Design review of the part built by this model. Coordinates are the model's own, in mm. A direction names the side the tool comes from. Give positions to 0.01 mm unless a question says otherwise; leave off trailing zeros. Loops run counter-clockwise (first coordinate to the right, second up) from the corner with the lowest first, then second, coordinate; pieces in that order, holes last.
Autodesk Inventor part; units mm, degrees
ref_plane "ABDECKKAPPE_XY" through (0, 0, 158) normal (0, 0, 1) x (1, 0, 0)
ref_plane "ABDECKKAPPE_YZ" through (0, 0, 158) normal (1, 0, 0) x (0, 1, 0)
ref_plane "ABDECKKAPPE_ZX" through (0, 0, 158) normal (0, 1, 0) x (0, 0, 1)
sketch "Sketch_1" plane through (0, 0, 0) normal (1, 0, 0) x (0, 0, -1)
  line L0 (0, 0) -> (-184, 0)
  line L1 (-184, 19.7) -> (-184, 17.75)
  line L2 (-184, 17.75) -> (-183.5, 17.25)
  line L3 (-183.5, 17.25) -> (-165, 17.25)
  line L4 (-165, 17.25) -> (-164.2489, 16)
  line L5 (-164.2489, 16) -> (-22.7511, 16)
  line L6 (-22.7511, 16) -> (-22, 17.25)
  line L7 (-22, 17.25) -> (-3, 17.25)
  line L8 (-3, 17.25) -> (-3, 18.5)
  line L9 (-3, 18.5) -> (0, 18.5)
  line L10 (0, 18.5) -> (0, 20)
  line L11 (0, 20) -> (-162.7709, 20)
  arc A0 (-163.2291, 20) -> (-162.7709, 20) centre (-163, 20.1) ccw
  line L12 (-163.2291, 20) -> (-183.7, 20)
  line L13 (-183.7, 20) -> (-184, 19.7)
revolve "Revolution1" add sketch "Sketch_1" angle 360 about axis through (0, 0, 0) along (0, 0, -1)
ref_plane "ABDECKKAPPE_XY" through (0, 0, 158) normal (0, 0, 1) x (1, 0, 0)
ref_plane "ABDECKKAPPE_YZ" through (0, 0, 158) normal (1, 0, 0) x (0, 1, 0)
ref_plane "ABDECKKAPPE_ZX" through (0, 0, 158) normal (0, 1, 0) x (0, 0, 1)
ref_plane "SCHUBSTANGE_XY" through (0, 0, 184) normal (0, 0, -1) x (1, 0, 0)
ref_plane "SCHUBSTANGE_YZ" through (0, 0, 184) normal (1, 0, 0) x (0, -1, 0)
ref_plane "SCHUBSTANGE_ZX" through (0, 0, 184) normal (0, -1, 0) x (0, 0, -1)
properties part number "SLZ_63_Schubstange#_274.5_1001"
Q1. Draft analysis for pull direction X (two halves, no side actions). For faces 3 (the face through (19.524, -4.336, 173.608)), 4 (the face through (-18, 6, 0)), 5 (the face through (5.181, 16.453, 174.12)), state which applies: pulls with the +X half, pulls with the -X half, needs draft (parallel to the pull), parting line crosses it, or undercut.
Results:
face 3: parting line crosses it
face 4: needs draft
face 5: undercut
Q2. Take a section at D-D (z = 25). Give the boundary of the cut face in (x, y).
Results:
outline: circle Ø40 at (0, 0); hole circle Ø32 at (0, 0)
Q3. Wall thickness on line 1 (X direction, y = 0, z = 51); line 2 (X direction, y = -0.5, z = 174); line 3 (Y direction, x = 8, z = 64): over which ranges is each line inside the solid? List them lowest first.
Results:
line 1: x = -20 to -16, 16 to 20
line 2: x = -19.99 to -17.24, 17.24 to 19.99
line 3: y = -18.33 to -13.86, 13.86 to 18.33
Q4. Insertion check: pin 1 (1.5 mm diameter, centred on x = -6.5, z = 73.5, fed in from +Y); pin 2 (8 mm diameter, centred on y = 7.5, z = 108.5, fed in from -X); pin 3 (6 mm diameter, centred on y = 3, z = 135, fed in from +X). Each pin has a flat end and moves straight along its axis. Give the tip position at first contact, or say it passes through.
Results:
pin 1: stops at y = 19.16
pin 2: stops at x = -19.69
pin 3: stops at x = 20
Q5. Tool access review of faces 1 (the face through (19.524, -4.336, 82.525)), 2 (the face through (17, 5, 3)): name each direction out of +Z, -Z, +X, -X, +Y, -Y from which nothing blocks a thin tool from reaching the whole face with its end or side.
Results:
face 1: +Z, -Z
face 2: -Z
Q6. Take a section at A-A (x = 0). Give the boundary of the cut face in (y, z), plus the area to 3 significant figures.
Results:
outline: (-20, 0) - (-18.5, 0) - (-18.5, 3) - (-17.25, 3) - (-17.25, 22) - (-16, 22.75) - (-16, 164.25) - (-17.25, 165) - (-17.25, 183.5) - (-17.75, 184) - (-19.7, 184) - (-20, 183.7) - (-20, 163.23) arc R0.25 cw to (-20, 162.77) - close; (16, 22.75) - (17.25, 22) - (17.25, 3) - (18.5, 3) - (18.5, 0) - (20, 0) - (20, 162.77) arc R0.25 cw to (20, 163.23) - (20, 183.7) - (19.7, 184) - (17.75, 184) - (17.25, 183.5) - (17.25, 165) - (16, 164.25) - close
area: 1,360 mm2
Q7. Take a section at C-C (z = 168.5). Give the boundary of the cut face in (x, y).
Results:
outline: circle Ø40 at (0, 0); hole circle Ø34.5 at (0, 0)
